Check sheet for the modelled part. Datum: model origin and axes. Units: mm. Face numbers are marked on the shaded views. A direction names the side the tool comes from. Round coordinates to 2 decimals unless told otherwise and drop trailing zeros. Write each loop counter-clockwise with the first axis right and the second up, starting at its lowest first coordinate (ties: lowest second). Pieces come first, ordered by that corner, then holes. Notation, with made-up numbers: (-10, 1) -> (45, 1) arc R34 cw to (45, 37) -> close; hole circle Ø11 at (20.25, -36). An arc over 180 degrees is marked (long way). Write item = value, one per line.
from build123d import *

# Parameters (mm, degrees)
SKETCH1_W                = 50
SKETCH1_H                = 50
BOSS_EXTRUDE1_DEPTH      = 50
CUT_EXTRUDE1_DEPTH       = 87.602540378
CUT_EXTRUDE2_DEPTH       = 87.602540378
CHAMFER1_SIZE            = 1.5
BOSS_EXTRUDE2_REACH      = 81.347
SKETCH11_W               = 0.5
SKETCH11_H               = 22
BOSS_EXTRUDE3_DEPTH      = 7
BOSS_EXTRUDE3_DEPTH_BACK = 10
SKETCH12_W               = 1
SKETCH12_H               = 7
SKETCH13_W               = 1.8
SKETCH13_H               = 1.8
CUT_EXTRUDE3_DEPTH       = 7


with BuildPart() as part:
    # Sketch1 → Boss-Extrude1 (new body)
    with BuildSketch(Plane.XY):
        with Locations((25, 25)):
            Rectangle(SKETCH1_W, SKETCH1_H)
    extrude(amount=BOSS_EXTRUDE1_DEPTH)

    # Sketch2 → Cut-Extrude1 (cut, through all)
    with BuildSketch(Plane.ZY):
        Polygon((45.443650814, 14), (54.556349186, 14), (61, 20.443650814), (61, 29.556349186), (54.556349186, 36), (45.443650814, 36), (39, 29.556349186), (39, 20.443650814), align=None)
        Polygon((36, 29.556349186), (29.556349186, 36), (20.443650814, 36), (14, 29.556349186), (14, 20.443650814), (20.443650814, 14), (29.556349186, 14), (36, 20.443650814), align=None)
    extrude(amount=-CUT_EXTRUDE1_DEPTH, mode=Mode.SUBTRACT)

    # Sketch10 → Cut-Extrude2 (cut, through all)
    with BuildSketch(Plane.XZ):
        Polygon((29.556349186, 36), (20.443650814, 36), (14, 29.556349186), (14, 20.443650814), (20.443650814, 14), (29.556349186, 14), (36, 20.443650814), (36, 29.556349186), align=None)
        Polygon((29.556349186, 39), (36, 45.443650814), (36, 54.556349186), (29.556349186, 61), (20.443650814, 61), (14, 54.556349186), (14, 45.443650814), (20.443650814, 39), align=None)
    extrude(amount=-CUT_EXTRUDE2_DEPTH, mode=Mode.SUBTRACT)

    # Chamfer1
    chamfer1_edges = [part.edges().sort_by_distance(p)[0] for p in [
        (50, 7, 50),
        (0, 7, 50),
        (50, 43, 50),
        (43, 14, 50),
        (7, 36, 50),
        (50, 36, 47.721825407),
        (50, 14, 47.721825407),
        (0, 14, 47.721825407),
        (0, 36, 47.721825407),
        (0, 32.778174593, 42.221825407),
        (0, 17.221825407, 42.221825407),
        (50, 17.221825407, 42.221825407),
        (50, 32.778174593, 42.221825407),
        (43, 50, 50),
        (7, 14, 50),
        (43, 36, 50),
        (43, 0, 50),
        (7, 50, 50),
        (36, 0, 47.721825407),
        (14, 0, 47.721825407),
        (17.221825407, 0, 42.221825407),
        (32.778174593, 0, 42.221825407),
        (14, 43, 50),
        (14, 50, 47.721825407),
        (14, 7, 50),
        (36, 50, 47.721825407),
        (36, 43, 50),
        (36, 7, 50),
        (17.221825407, 50, 42.221825407),
        (32.778174593, 50, 42.221825407),
        (0, 43, 50),
        (25, 50, 0),
        (50, 25, 0),
        (25, 0, 0),
        (0, 25, 0),
        (7, 0, 50),
        (0, 50, 25),
        (50, 50, 25),
        (50, 0, 25),
        (0, 0, 25),
    ]]
    chamfer(chamfer1_edges, length=CHAMFER1_SIZE)

    # Boss-Extrude2: up to this face of the body (flat: up to its plane)
    boss_extrude2_end = Plane(part.part.faces().sort_by_distance((25, 25, 39))[0])
    # Sketch11 → Boss-Extrude2 (add, up to the picked face)
    with BuildSketch(Plane.XY.offset(14), mode=Mode.PRIVATE) as boss_extrude2_sk1:
        with Locations((36.25, 25)):
            Rectangle(SKETCH11_W, SKETCH11_H)
    boss_extrude2_tool1 = split(extrude(boss_extrude2_sk1.sketch, amount=BOSS_EXTRUDE2_REACH, mode=Mode.PRIVATE), bisect_by=boss_extrude2_end, keep=Keep.BOTH, mode=Mode.PRIVATE)
    # Sketch11 → Boss-Extrude2 (add, up to the picked face)
    with BuildSketch(Plane.XY.offset(14), mode=Mode.PRIVATE) as boss_extrude2_sk2:
        with Locations((13.75, 25)):
            Rectangle(SKETCH11_W, SKETCH11_H)
    boss_extrude2_tool2 = split(extrude(boss_extrude2_sk2.sketch, amount=BOSS_EXTRUDE2_REACH, mode=Mode.PRIVATE), bisect_by=boss_extrude2_end, keep=Keep.BOTH, mode=Mode.PRIVATE)
    # Sketch11 → Boss-Extrude2 (add, up to the picked face)
    with BuildSketch(Plane.XY.offset(14), mode=Mode.PRIVATE) as boss_extrude2_sk3:
        with Locations((49.25, 25)):
            Rectangle(SKETCH11_W, SKETCH11_H)
    boss_extrude2_tool3 = split(extrude(boss_extrude2_sk3.sketch, amount=BOSS_EXTRUDE2_REACH, mode=Mode.PRIVATE), bisect_by=boss_extrude2_end, keep=Keep.BOTH, mode=Mode.PRIVATE)
    # Sketch11 → Boss-Extrude2 (add, up to the picked face)
    with BuildSketch(Plane.XY.offset(14), mode=Mode.PRIVATE) as boss_extrude2_sk4:
        with Locations((0.75, 25)):
            Rectangle(SKETCH11_W, SKETCH11_H)
    boss_extrude2_tool4 = split(extrude(boss_extrude2_sk4.sketch, amount=BOSS_EXTRUDE2_REACH, mode=Mode.PRIVATE), bisect_by=boss_extrude2_end, keep=Keep.BOTH, mode=Mode.PRIVATE)
    add(boss_extrude2_tool1.solids().sort_by(Axis((36.25, 25, 14), (0, 0, 1)))[0])
    add(boss_extrude2_tool2.solids().sort_by(Axis((13.75, 25, 14), (0, 0, 1)))[0])
    add(boss_extrude2_tool3.solids().sort_by(Axis((49.25, 25, 14), (0, 0, 1)))[0])
    add(boss_extrude2_tool4.solids().sort_by(Axis((0.75, 25, 14), (0, 0, 1)))[0])

    # Sketch12 → Boss-Extrude3 (add, two sides: drawn at the far end of the back side and taken through both)
    with BuildSketch(Plane.XY.offset(50).offset(-BOSS_EXTRUDE3_DEPTH_BACK)):
        with Locations((49.5, 7)):
            Rectangle(SKETCH12_W, SKETCH12_H)
    extrude(amount=BOSS_EXTRUDE3_DEPTH + BOSS_EXTRUDE3_DEPTH_BACK)

    # Sketch13 → Cut-Extrude3 (cut)
    with BuildSketch(Plane(origin=(50, 0, 0), x_dir=(0, 0, -1), z_dir=(1, 0, 0))):
        with Locations((-53.6, 7)):
            Rectangle(SKETCH13_W, SKETCH13_H)
    extrude(amount=-CUT_EXTRUDE3_DEPTH, mode=Mode.SUBTRACT)


solid = part.part
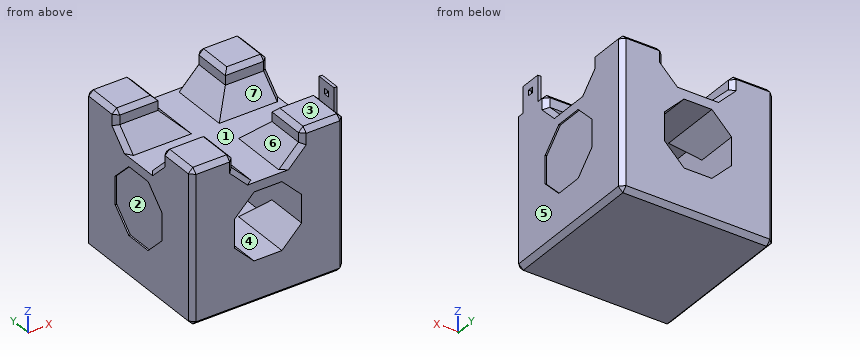
(1) Sectioned sample at B-B on z = 27. Enter the section's corners in (x, y), then the cut area to 4 significant figures.
Worked answers:
outline = (0, 1.5) -> (1.5, 0) -> (14, 0) -> (14, 50) -> (1.5, 50) -> (0, 48.5) -> (0, 36) -> (0.5, 36) -> (0.5, 14) -> (0, 14) -> close; (36, 0) -> (48.5, 0) -> (50, 1.5) -> (50, 14) -> (49.5, 14) -> (49.5, 36) -> (50, 36) -> (50, 48.5) -> (48.5, 50) -> (36, 50) -> close; hole (1, 14) -> (13.5, 14) -> (13.5, 36) -> (1, 36) -> close; hole (36.5, 14) -> (49, 14) -> (49, 36) -> (36.5, 36) -> close
area = 823.5 mm²
(2) Sectioned sample at D-D on z = 41.5. Enter the section's corners in (x, y), then the cut area to 3 significant figures.
Worked answers:
outline = (0, 1.5) -> (1.5, 0) -> (15.82, 0) -> (17.94, 1.5) -> (17.94, 17.94) -> (1.5, 17.94) -> (0, 15.82) -> close; (0, 34.18) -> (1.5, 32.06) -> (17.94, 32.06) -> (17.94, 48.5) -> (15.82, 50) -> (1.5, 50) -> (0, 48.5) -> close; (32.06, 1.5) -> (34.18, 0) -> (48.5, 0) -> (50, 1.5) -> (50, 15.82) -> (48.5, 17.94) -> (32.06, 17.94) -> close; (32.06, 32.06) -> (48.5, 32.06) -> (50, 34.18) -> (50, 48.5) -> (48.5, 50) -> (34.18, 50) -> (32.06, 48.5) -> close
area = 1,270 mm²
(3) Access from +Z, -Z, +X, -X, +Y, -Y to the whole of each face (thin tool, end or side, straight path). Record for the marked faces 1, 2, 3 and 4.
Worked answers:
face_1 = +Z
face_2 = -X
face_3 = +Z, -X, +Y, -Y
face_4 = none
(4) Go/stop test with flat-tipped pins: P1, Ø8, axis at x = 28, z = 21, coming from the -Y side; P2, Ø12, axis at x = 8.5, y = 43.5, coming from the +Z side; P3, Ø0.6, axis at x = 0.5, z = 27, coming from the +Y side; P4, Ø1.5, axis at y = 31, z = 17, coming from the -X side. Record where each tip stops, or that it passes through.
Worked answers:
P1 = through
P2 = 50
P3 = 49.3
P4 = 0.5
(5) Release check for a two-part mould opening along X. For the marked faces 5, 6 and 7 record: pulls with the +X half, pulls with the -X half, needs draft (parallel to the pull), parting line crosses it, or undercut.
Worked answers:
face_5 = pulls with the +X half
face_6 = undercut
face_7 = needs draft
(6) Material ranges on L1, parallel to X at y = 18.5, z = 32; L2, parallel to Y at x = 45, z = 49; L3, parallel to Z at x = 18.5, y = 28, recorded low to high. Write a range as [from, to].
Worked answers:
L1 = [0.5, 1], [13.5, 14], [36, 36.5], [49, 49.5]
L2 = [0.5, 13.5], [36.5, 49.5]
L3 = [0, 14], [36, 39]
(7) Sectioned sample at A-A on y = 40. Enter the section's corners in (x, z), then the cut area to 3 significant figures.
Worked answers:
outline = (0, 1.5) -> (1.5, 0) -> (48.5, 0) -> (50, 1.5) -> (50, 48.5) -> (48.5, 50) -> (37.5, 50) -> (36, 48.5) -> (36, 45.44) -> (29.56, 39) -> (20.44, 39) -> (14, 45.44) -> (14, 48.5) -> (12.5, 50) -> (1.5, 50) -> (0, 48.5) -> close; hole (14, 20.44) -> (20.44, 14) -> (29.56, 14) -> (36, 20.44) -> (36, 29.56) -> (29.56, 36) -> (20.44, 36) -> (14, 29.56) -> close
area = 1,890 mm²
(8) Sectioned sample at C-C on x = 27. Enter the section's corners in (y, z), then the cut area to 3 significant figures.
Worked answers:
outline = (0, 1.5) -> (1.5, 0) -> (48.5, 0) -> (50, 1.5) -> (50, 14) -> (0, 14) -> close; (0, 36) -> (50, 36) -> (50, 39) -> (0, 39) -> close
area = 848 mm²
